from build123d import *

# Parameters (mm, degrees)
SKETCH_1_W          = 6
SKETCH_1_H          = 6
EXTRUDE_1_DEPTH     = 22
SKETCH_3_R          = 1.55
CUT_EXTRUDE_1_DEPTH = 44
SKETCH_6_R          = 1.55
CUT_EXTRUDE_2_DEPTH = 10


with BuildPart() as part:
    # 草图1 → 凸台-拉伸1 (new, symmetric)
    with BuildSketch(Plane.XY):
        Rectangle(SKETCH_1_W, SKETCH_1_H)
    extrude(amount=EXTRUDE_1_DEPTH, both=True)

    # 草图3 → 切除-拉伸1 (cut)
    with BuildSketch(Plane(origin=(3, 0, 0), x_dir=(0, 0, -1), z_dir=(1, 0, 0))):
        with Locations(Location((-17.5, 0, 0), (0, 0, 90))):
            Circle(SKETCH_3_R)
        with Locations(Location((17.5, 0, 0), (0, 0, 90))):
            Circle(SKETCH_3_R)
    extrude(amount=-CUT_EXTRUDE_1_DEPTH, mode=Mode.SUBTRACT)

    # 草图6 → 切除-拉伸2 (cut)
    with BuildSketch(Plane(origin=(0, 3, 0), x_dir=(1, 0, 0), z_dir=(0, 1, 0))):
        with Locations(Location((-0.320508076, -10, 0), (0, 0, 270))):
            Circle(SKETCH_6_R)
        with Locations(Location((-0.320508076, 10, 0), (0, 0, 270))):
            Circle(SKETCH_6_R)
    extrude(amount=-CUT_EXTRUDE_2_DEPTH, mode=Mode.SUBTRACT)


solid = part.part
The listing builds one solid part. Answer for the finished solid, in the listing's coordinates (mm). Coordinates: 2 decimals unless noted, no trailing zeros. Loops run counter-clockwise (first coordinate to the right, second up) from the corner with the lowest first, then second, coordinate; pieces in that order, holes last. Notation, with made-up numbers: (-18, 67.5) -> (37, 67.5) arc R33 ccw to (37, 95.5) -> close; hole circle Ø11 at (36, 40.5). An arc over 180 degrees is marked (long way). Answer in a Markdown table with one row per item. Add a question column.
1. Determine the mould class of faces 1 (the flat face through (0, 0, 22)), 2 (the cylindrical face through (-1.3, 0, 8.8)), 3 (the flat face through (0, -3, 0)), 4 (the cylindrical face through (0.042, -0.202, 19.037)) for opening direction Z: +Z half, -Z half, draft (parallel to the pull), parting line (faces both ways), or undercut.
2. The part is cut by section D-D, the plane z = -11. Write down the section's boundary in (x, y).
3. Consider line 1 (Z direction, x = 0.3, y = 0); line 2 (Z direction, x = 0.8, y = 0); line 3 (Z direction, x = 0.5, y = -2.2). Determine where each line is inside the solid, lowest interval first. Write a range as [from, to].
4. The part is cut by section A-A, the plane z = 17.5. Write down the section's boundary in (x, y).
5. The part is cut by section B-B, the plane y = 0.1. Write down the section's boundary in (x, z), then the cut area to 3 significant figures.
6. The part is cut by section C-C, the plane x = -0.7. Write down the section's boundary in (y, z).
Answer below:
| question | item | result |
|---|---|---|
| 1 | face 1 | +Z half |
| 1 | face 2 | undercut |
| 1 | face 3 | draft |
| 1 | face 4 | undercut |
| 2 | outline | (-3, -3) -> (-1.5, -3) -> (-1.5, 3) -> (-3, 3) -> close; (0.86, -3) -> (3, -3) -> (3, 3) -> (0.86, 3) -> close |
| 3 | line 1 | [-22, -19.05], [-15.95, -11.42], [-8.58, 8.58], [11.42, 15.95], [19.05, 22] |
| 3 | line 2 | [-22, -19.05], [-15.95, -11.07], [-8.93, 8.93], [11.07, 15.95], [19.05, 22] |
| 3 | line 3 | [-22, -11.32], [-8.68, 8.68], [11.32, 22] |
| 4 | outline | (-3, -3) -> (3, -3) -> (3, -1.55) -> (-3, -1.55) -> close; (-3, 1.55) -> (3, 1.55) -> (3, 3) -> (-3, 3) -> close |
| 5 | outline | (-3, -22) -> (3, -22) -> (3, -19.05) -> (-3, -19.05) -> close; (-3, -15.95) -> (3, -15.95) -> (3, 15.95) -> (-3, 15.95) -> close; (-3, 19.05) -> (3, 19.05) -> (3, 22) -> (-3, 22) -> close; hole circle Ø3.1 at (-0.32, -10); hole circle Ø3.1 at (-0.32, 10) |
| 5 | area | 212 mm2 |
| 6 | outline | (-3, -22) -> (3, -22) -> (3, -11.5) -> (-3, -11.5) -> close; (-3, -8.5) -> (3, -8.5) -> (3, 8.5) -> (-3, 8.5) -> close; (-3, 11.5) -> (3, 11.5) -> (3, 22) -> (-3, 22) -> close; hole circle Ø3.1 at (0, -17.5); hole circle Ø3.1 at (0, 17.5) |
